Here's how the part is built. I have some questions about the finished solid (model axes, mm). A direction names the side the tool comes from. Give positions to 0.01 mm unless a question says otherwise; leave off trailing zeros. Loops run counter-clockwise (first coordinate to the right, second up) from the corner with the lowest first, then second, coordinate; pieces in that order, holes last. Notation, with made-up numbers: (71, 53) -> (109, 53) arc R10 cw to (109, 63) -> close; hole circle Ø9 at (0.25, 70). An arc over 180 degrees is marked (long way). Answer in a Markdown table with one row per item. Add a question column.
Item 1: If I drill on line 1 (X direction, y = 14.75, z = -8); line 2 (X direction, y = 4, z = -7); line 3 (Y direction, x = -6.5, z = -8.45), over which ranges is the centre line in solid material (lowest first)?
Item 2: If we section it at A-A (y = 6.5): Write out the boundary of the cut face in (x, z), then the cut area to 3 significant figures.
Item 3: If we section it at B-B (x = -4.75): Write out the boundary of the cut face in (y, z), then the cut area to 3 significant figures.
Item 4: If we section it at D-D (y = 15.25): Write out the boundary of the cut face in (x, z).
Item 5: Which directions (+Z, -Z, +X, -X, +Y, -Y) give clear straight access to the entire face, cutting with the end or side of a thin tool? Please do faces 1 (the face through (0.914, 16, -8)), 2 (the face through (-3, 21.617, -8)), 3 (the face through (-7.086, 16, -8)).
Item 6: For P1, Ø1, axis at y = 9, z = -7.5, coming from the -X side; P2, Ø1, axis at x = 0.5, z = -8, coming from the -Y side; P3, Ø0.6, axis at y = 17.5, z = -7, coming from the +X side, each with a flat end and sliding along its axis, tell me the tip position at first contact or that it passes through.
Item 7: If we section it at C-C (z = -7.5): Write out the boundary of the cut face in (x, y).
Autodesk Inventor part; units mm, degrees
ref_plane "Work Plane2" through (-10, -10, -4.4) normal (0, 0, 1) x (1, 0, 0)
ref_plane "YZ Plane" through (0, 0, 0) normal (1, 0, 0) x (0, 1, 0)
ref_plane "XZ Plane" through (0, 0, 0) normal (0, 1, 0) x (-1, 0, 0)
ref_plane "Work Plane1" through (0, 0, -6.6) normal (0, 0, -1) x (-1, 0, 0)
sketch "Sketch1" plane through (0, 0, -6.6) normal (0, 0, -1) x (-1, 0, 0)
  circle A0 centre (3.0857, 5.1173) radius 10
  line L0 (-6.9143, 5.1173) -> (-6.9143, 18.1173)
  line L1 (-6.9143, 18.1173) -> (13.0857, 18.1173)
  line L2 (13.0857, 18.1173) -> (13.0857, 5.1173)
  circle A1 centre (0, 0) radius 5
  point P0 (0, 0)
  dimension "d24" = 13
  dimension "d25" = 20
ref_plane "Work Plane2" through (-10, -10, -4.4) normal (0, 0, 1) x (1, 0, 0)
extrude "Extrusion1" add sketch "Sketch1" along normal blind 2 contours A0 A1 | A0 L0 L1 L2 | A0 A1 picked at (6.1055, 10.6249) picked at (0.8611, -2.5748)
sketch "Sketch9" plane through (0, 0, -8.6) normal (0, 0, -1) x (-1, 0, 0)
  circle A0 centre (3.0857, 5.1173) radius 5 construction
  arc A1 (-6.9143, 5.1173) -> (13.0857, 5.1173) centre (3.0857, 5.1173) ccw
  circle A2 centre (3.0857, 5.1173) radius 3.75
  dimension "d43" = 7.5
extrude "Extrusion6" cut sketch "Sketch9" against normal up to surface (2 mm away)
sketch "Sketch10" plane through (0, 0, -8.6) normal (0, 0, -1) x (-1, 0, 0)
  arc A0 (-6.9143, 5.1173) -> (13.0857, 5.1173) centre (3.0857, 5.1173) ccw
  line L0 (3.0857, -4.8827) -> (3.0857, -2.8827)
  line L1 (3.0857, -2.8827) -> (4.5857, -2.8827)
  line L2 (4.5857, -2.8827) -> (3.0857, -2.8827)
  line L3 (-2.1325, -2.8827) -> (-2.1325, -5.7607)
  line L4 (4.5857, -2.8827) -> (4.5857, -3.3119)
  line L5 (-2.1325, -5.7607) -> (-2.1325, -7.2943)
  line L6 (4.5857, -3.3119) -> (4.5857, -2.7408)
  line L7 (-4, 15) -> (-4, 13) construction
  line L8 (4, 13) -> (4, 15) construction
  line L9 (13.0857, 18.1173) -> (-6.9143, 18.1173)
  line L10 (-6.9143, 18.1173) -> (13.0857, 18.1173)
  line L11 (-6.9143, 18.1173) -> (-6.9143, 5.1173)
  line L12 (13.0857, 18.1173) -> (13.0857, 5.1173)
  arc A1 (-6.9143, 5.1173) -> (13.0857, 5.1173) centre (3.0857, 5.1173) ccw
  circle A2 centre (3.0857, 5.1173) radius 6.5
  line L13 (3.0857, 5.1173) -> (3.0857, 11.6173) construction
  line L14 (3.0857, 11.6173) -> (7.0857, 11.6173)
  line L15 (7.0857, 11.6173) -> (3.0857, 11.6173)
  line L16 (3.0857, 11.6173) -> (-0.9143, 11.6173)
  line L17 (-0.9143, 10.2408) -> (-0.9143, 18.1173)
  line L18 (-0.9143, 18.1173) -> (7.0857, 18.1173)
  line L19 (7.0857, 18.1173) -> (7.0857, 10.2408)
  point P0 (5.6921, -0.9362)
  dimension "d31" = 2
  dimension "d37" = 1.5
  dimension "d44" = 4
  dimension "d45" = 4
extrude "Extrusion8" cut sketch "Sketch10" against normal up to next contours A0 L11 L9 L17 A2 L19 L12
sketch "Sketch11" plane through (0, 0, -8.6) normal (0, 0, -1) x (-1, 0, 0)
  line L0 (7.0857, 18.1173) -> (-0.9143, 18.1173)
  line L1 (7.0857, 18.1173) -> (7.0857, 21.6173)
  line L2 (7.0857, 21.6173) -> (-0.9143, 21.6173)
  line L3 (-0.9143, 21.6173) -> (-0.9143, 18.1173)
  point P0 (0, 0)
  dimension "d46" = 3.5
extrude "Extrusion9" add sketch "Sketch11" against normal up to surface (2 mm away)
Recorded:
| question | item | result |
|---|---|---|
| 1 | line 1 | x = -7.09 to 0.91 |
| 1 | line 2 | x = -9.49 to -6.67, 0.49 to 3.32 |
| 1 | line 3 | y = -0.41 to 3.57, 6.67 to 21.62 |
| 2 | outline | (-9.44, -8.6) -> (-6.57, -8.6) -> (-6.57, -6.6) -> (-9.44, -6.6) -> close; (0.4, -8.6) -> (3.27, -8.6) -> (3.27, -6.6) -> (0.4, -6.6) -> close |
| 2 | area | 11.5 mm^2 |
| 3 | outline | (-1.17, -8.6) -> (1.76, -8.6) -> (1.76, -6.6) -> (-1.17, -6.6) -> close; (8.48, -8.6) -> (21.62, -8.6) -> (21.62, -6.6) -> (8.48, -6.6) -> close |
| 3 | area | 32.1 mm^2 |
| 4 | outline | (-7.09, -8.6) -> (0.91, -8.6) -> (0.91, -6.6) -> (-7.09, -6.6) -> close |
| 5 | face 1 | +Z, -Z, +X, +Y |
| 5 | face 2 | +Z, -Z, +X, -X, +Y |
| 5 | face 3 | +Z, -Z, -X, +Y |
| 6 | P1 | stops at x = -8.64 |
| 6 | P2 | stops at y = -0.6 |
| 6 | P3 | stops at x = 0.91 |
| 7 | outline | (-7.09, 10.24) arc R6.5 ccw (long way) to (0.91, 10.24) -> (0.91, 21.62) -> (-7.09, 21.62) -> close; hole circle Ø7.5 at (-3.09, 5.12) |
